The listing builds one solid part. Answer for the finished solid, in the listing's coordinates (mm). Round coordinates to 2 decimals unless told otherwise and drop trailing zeros. Order: outer loops, then holes, each group sorted by start corner. A loop starts at its lowest first (then second) coordinate and runs counter-clockwise, first axis right, second up. Notation, with made-up numbers: (61, 84) - (97, 84) arc R17 cw to (97, 116) - close; hole circle Ø11 at (27.25, -1). An arc over 180 degrees is marked (long way). One line per item, written item: value. Start each with the question number.
1. For a pull along Y with two mould halves and no side action, classify faces 1 (the flat face through (50, 6, 3.175)), 2 (the cylindrical face through (67.563, 7.742, 1.565)), 3 (the flat face through (50, 12.7, 2)) as released by +Y, released by -Y, zero draft, split by the parting line, or undercut.
2. Section B-B, the plane x = 54 is taken. Give the vertices of the cut face in (y, z) (3 decimals).
3. Section A-A, the plane z = 1.95 is taken. Count the separate pieces of the cut face and the enclosed holes in it, then the cut area to 3 significant figures.
4. A flat-ended cylindrical pin translates along its axis: P1, Ø4.5, axis at x = 34.925, y = 6.35, coming from the -Z side. Find the tip coordinate at first contact, or state that the pin passes through.
5. Section D-D, the plane x = 40.5 is taken. Give the vertices of the cut face in (y, z) (3 decimals).
6. Straight lines are drawn through the part: line 1 (Y direction, x = 60.5, z = 1.1); line 2 (Y direction, x = 40.5, z = 1.65). For each, find the intervals that lie inside material, in ascending order.
from build123d import *

# Parameters (mm, degrees)
SKETCH1_W               = 101.6
SKETCH1_H               = 12.7
BOSS_EXTRUDE3_DEPTH     = 3.175
SKETCH2_R               = 1.651
CUT_EXTRUDE1_DEPTH      = 127
CUT_EXTRUDE1_DEPTH_BACK = 127


with BuildPart() as part:
    # Sketch1 → Boss-Extrude3 (new body)
    with BuildSketch(Plane.XY):
        with Locations((50.8, 6.35)):
            Rectangle(SKETCH1_W, SKETCH1_H)
    extrude(amount=BOSS_EXTRUDE3_DEPTH)

    # Sketch2 → Cut-Extrude1 (cut, two sides)
    with BuildSketch(Plane.XY) as cut_extrude1_sk:
        with Locations((3.175, 6.35)):
            Circle(SKETCH2_R)
        with Locations((9.525, 6.35)):
            Circle(SKETCH2_R)
        with Locations((15.875, 6.35)):
            Circle(SKETCH2_R)
        with Locations((22.225, 6.35)):
            Circle(SKETCH2_R)
        with Locations((28.575, 6.35)):
            Circle(SKETCH2_R)
        with Locations((34.925, 6.35)):
            Circle(SKETCH2_R)
        with Locations((41.275, 6.35)):
            Circle(SKETCH2_R)
        with Locations((47.625, 6.35)):
            Circle(SKETCH2_R)
        with Locations((53.975, 6.35)):
            Circle(SKETCH2_R)
        with Locations((60.325, 6.35)):
            Circle(SKETCH2_R)
        with Locations((66.675, 6.35)):
            Circle(SKETCH2_R)
        with Locations((73.025, 6.35)):
            Circle(SKETCH2_R)
        with Locations((79.375, 6.35)):
            Circle(SKETCH2_R)
        with Locations((85.725, 6.35)):
            Circle(SKETCH2_R)
        with Locations((92.075, 6.35)):
            Circle(SKETCH2_R)
        with Locations((98.425, 6.35)):
            Circle(SKETCH2_R)
    extrude(amount=CUT_EXTRUDE1_DEPTH, mode=Mode.SUBTRACT)
    extrude(cut_extrude1_sk.sketch, amount=-CUT_EXTRUDE1_DEPTH_BACK, mode=Mode.SUBTRACT)


solid = part.part
Answer list:
1. face 1: zero draft
1. face 2: undercut
1. face 3: released by +Y
2. outline: (0, 0) - (4.699, 0) - (4.699, 3.175) - (0, 3.175) - close; (8.001, 0) - (12.7, 0) - (12.7, 3.175) - (8.001, 3.175) - close
3. separate pieces: 1
3. enclosed holes: 16
3. area: 1,150 mm²
4. P1: stops at z = 0
5. outline: (0, 0) - (4.892, 0) - (4.892, 3.175) - (0, 3.175) - close; (7.808, 0) - (12.7, 0) - (12.7, 3.175) - (7.808, 3.175) - close
6. line 1: y = 0 to 4.71, 7.99 to 12.7
6. line 2: y = 0 to 4.89, 7.81 to 12.7
